For this review, take the finished solid that the model builds, in its own axes (mm). Face numbers are marked on the shaded views. A direction names the side the tool comes from. Give positions to 0.01 mm unless a question says otherwise; leave off trailing zeros. Order: outer loops, then holes, each group sorted by start corner. A loop starts at its lowest first (then second) coordinate and runs counter-clockwise, first axis right, second up. Notation, with made-up numbers: M -13,83 L 40,83 A35 cw 40,122 Z; hole C -0.5,-18.75 d6. An arc over 180 degrees is marked long. Answer as CSV lines item,"result". Start each with the question number.
1. Clearance check with flat-ended pins moving along their axes: P1, Ø21, axis at x = 7, z = -10.5, coming from the -Y side; P2, Ø6, axis at x = 6.5, y = 45.5, coming from the +Z side; P3, Ø10, axis at x = 39.5, y = 15, coming from the +Z side. State where each tip first meets the part, or that it passes through.
2. For line 1 along X through (y, z) = (13.5, 0); line 2 along X through (y, z) = (27.55, 0); line 3 along Y through (x, z) = (-31.5, 0), list the stretches that pass through material, from the lowest coordinate up.
3. Machinability: for the marked faces 1, 2 and 3, which of the approach directions +Z, -Z, +X, -X, +Y, -Y give a long, thin tool a straight path to every point of the face, cutting with its end or side? Answer none if there is none.
4. We need section B-B, the plane y = 13. Give the boundary of the cut face in (x, z).
5. Mouldability with a two-part tool opening along Z and no side actions: class the marked faces 4, 5 and 6 as pulls with the +Z half, pulls with the -Z half, needs draft (parallel to the pull), parting line crosses it, or undercut.
6. We need section A-A, the plane y = 69. Give the boundary of the cut face in (x, z), and give its area (3 significant figures).
from build123d import *


with BuildPart() as part:
    # Esquisse1 → Révolution1 (revolve)
    with BuildSketch(Plane.XY, mode=Mode.PRIVATE) as r_volution1_sk:
        with BuildLine():
            Line((33, 94.535053287), (33, 51.422205102))
            ThreePointArc((33, 51.422205102), (34.607695155, 45.422205102), (39, 41.029900256))
            Line((39, 41.029900256), (57, 30.637595411))
            ThreePointArc((57, 30.637595411), (59.196152423, 28.441442988), (60, 25.441442988))
            Line((60, 25.441442988), (60, 19.535053287))
            Line((60, 19.535053287), (59, 19.535053287))
            Line((59, 19.535053287), (59, 17.535053287))
            Line((59, 17.535053287), (60, 17.535053287))
            Line((60, 17.535053287), (60, 2.535053287))
            Line((60, 2.535053287), (59, 1.535053287))
            Line((59, 1.535053287), (57, 1.535053287))
            Line((57, 1.535053287), (57, 6.535053287))
            Line((57, 6.535053287), (49, 6.535053287))
            Line((49, 6.535053287), (49, 24.535053287))
            Line((49, 24.535053287), (55, 24.535053287))
            Line((55, 24.535053287), (55, 27.035053287))
            Line((55, 27.035053287), (50, 27.035053287))
            Line((50, 27.035053287), (50, 29.035053287))
            Line((50, 29.035053287), (49.01666888, 29.035053287))
            ThreePointArc((49.01666888, 29.035053287), (48.71714205, 29.953920875), (48.021719707, 30.625055533))
            Line((48.021719707, 30.625055533), (38.852533252, 35.9188878))
            ThreePointArc((38.852533252, 35.9188878), (37.136356036, 36.054212208), (35.950790389, 34.806009088))
            Line((35.950790389, 34.806009088), (35, 31.885724321))
            Line((35, 31.885724321), (28, 31.885724321))
            Line((28, 31.885724321), (27, 32.885724321))
            Line((27, 32.885724321), (27, 85.035053287))
            Line((27, 85.035053287), (22.5, 85.035053287))
            Line((22.5, 85.035053287), (21.5, 86.035053287))
            Line((21.5, 86.035053287), (21.5, 101.535053287))
            Line((21.5, 101.535053287), (32, 101.535053287))
            Line((32, 101.535053287), (32, 94.535053287))
            Line((32, 94.535053287), (33, 94.535053287))
        make_face()
    revolve(r_volution1_sk.sketch.rotate(Axis((0, 108.46930196, 0), (0, -1, 0)), 90), axis=Axis((0, 108.46930196, 0), (0, -1, 0)))  # turned: the seam where the file's is


solid = part.part
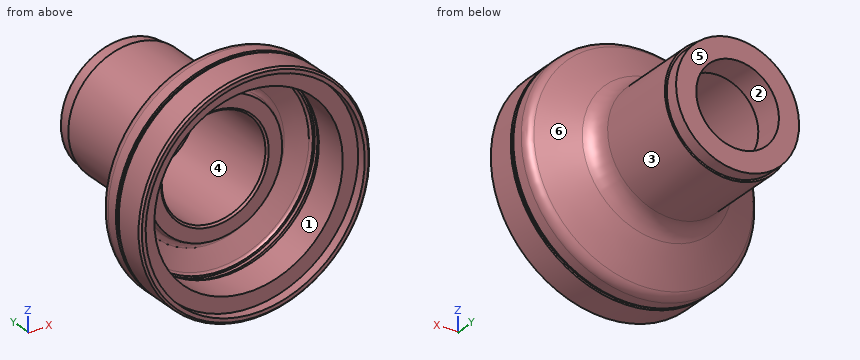
Result set:
1,P1,"y = 85.04"
1,P2,"z = 36.44"
1,P3,"z = 49.09"
2,line 1,"-60 to -49, 49 to 60"
2,line 2,"-59.62 to -50, 50 to 59.62"
2,line 3,"31.89 to 101.54"
3,face 1,"-Y"
3,face 2,"+Y, -Y"
3,face 3,"+Y"
4,outline,"C 0,0 d120; hole C 0,0 d98"
5,face 4,"undercut"
5,face 5,"needs draft"
5,face 6,"parting line crosses it"
6,outline,"C 0,0 d66; hole C 0,0 d54"
6,area,"1,130 mm2"
